from build123d import *

# Parameters (mm, degrees)
SKETCH_1_R      = 1.75
EXTRUDE_1_DEPTH = 3
FILLET_3_R      = 5


with BuildPart() as part:
    # 草图1 → 凸台-拉伸1 (new body)
    with BuildSketch(Plane(origin=(0, 0, 0), x_dir=(1, 0, 0), z_dir=(0, 1, 0))):
        with BuildLine():
            Line((-27.5, -18.562205506), (-37.85023308, -27.436866757))
            ThreePointArc((-37.85023308, -27.436866757), (-39.59101252, -31.447551796), (-37.512145027, -35.293876989))
            Line((-37.512145027, -35.293876989), (-26.035533906, -43.535533906))
            ThreePointArc((-26.035533906, -43.535533906), (-24.413417162, -44.619397663), (-22.5, -45))
            Line((-22.5, -45), (-22.5, -54))
            ThreePointArc((-22.5, -54), (-21.914213562, -55.414213562), (-20.5, -56))
            Line((-20.5, -56), (-16.5, -56))
            ThreePointArc((-16.5, -56), (-15.085786438, -55.414213562), (-14.5, -54))
            Line((-14.5, -54), (-14.5, -45))
            Line((-14.5, -45), (14.5, -45))
            Line((14.5, -45), (14.5, -54))
            ThreePointArc((14.5, -54), (15.085786438, -55.414213562), (16.5, -56))
            Line((16.5, -56), (20.5, -56))
            ThreePointArc((20.5, -56), (21.914213562, -55.414213562), (22.5, -54))
            Line((22.5, -54), (22.5, -45))
            ThreePointArc((22.5, -45), (24.413417162, -44.619397663), (26.035533906, -43.535533906))
            Line((26.035533906, -43.535533906), (37.512145027, -35.293876989))
            ThreePointArc((37.512145027, -35.293876989), (39.59101252, -31.447551796), (37.85023308, -27.436866757))
            Line((37.85023308, -27.436866757), (27.5, -18.562205506))
            Line((27.5, -18.562205506), (27.5, 18.562205506))
            Line((27.5, 18.562205506), (37.85023308, 27.436866757))
            ThreePointArc((37.85023308, 27.436866757), (39.59101252, 31.447551796), (37.512145027, 35.293876989))
            Line((37.512145027, 35.293876989), (26.035533906, 43.535533906))
            ThreePointArc((26.035533906, 43.535533906), (24.413417162, 44.619397663), (22.5, 45))
            Line((22.5, 45), (22.5, 54))
            ThreePointArc((22.5, 54), (21.914213562, 55.414213562), (20.5, 56))
            Line((20.5, 56), (16.5, 56))
            ThreePointArc((16.5, 56), (15.085786438, 55.414213562), (14.5, 54))
            Line((14.5, 54), (14.5, 45))
            Line((14.5, 45), (-14.5, 45))
            Line((-14.5, 45), (-14.5, 54))
            ThreePointArc((-14.5, 54), (-15.085786438, 55.414213562), (-16.5, 56))
            Line((-16.5, 56), (-20.5, 56))
            ThreePointArc((-20.5, 56), (-21.914213562, 55.414213562), (-22.5, 54))
            Line((-22.5, 54), (-22.5, 45))
            ThreePointArc((-22.5, 45), (-24.413417162, 44.619397663), (-26.035533906, 43.535533906))
            Line((-26.035533906, 43.535533906), (-37.512145027, 35.293876989))
            ThreePointArc((-37.512145027, 35.293876989), (-39.59101252, 31.447551796), (-37.85023308, 27.436866757))
            Line((-37.85023308, 27.436866757), (-27.5, 18.562205506))
            Line((-27.5, 18.562205506), (-27.5, -18.562205506))
        make_face()
        with Locations((-22.5, -40)):
            Circle(SKETCH_1_R, mode=Mode.SUBTRACT)
        with Locations((22.5, 40)):
            Circle(SKETCH_1_R, mode=Mode.SUBTRACT)
        with Locations((-35, -31.25)):
            Circle(SKETCH_1_R, mode=Mode.SUBTRACT)
        with Locations((-18.5, -49)):
            Circle(SKETCH_1_R, mode=Mode.SUBTRACT)
        with Locations((18.5, -49)):
            Circle(SKETCH_1_R, mode=Mode.SUBTRACT)
        with Locations((-35, 31.25)):
            Circle(SKETCH_1_R, mode=Mode.SUBTRACT)
        with Locations((35, -31.25)):
            Circle(SKETCH_1_R, mode=Mode.SUBTRACT)
        with Locations((-18.5, 49)):
            Circle(SKETCH_1_R, mode=Mode.SUBTRACT)
        with Locations((35, 31.25)):
            Circle(SKETCH_1_R, mode=Mode.SUBTRACT)
        with Locations((18.5, 49)):
            Circle(SKETCH_1_R, mode=Mode.SUBTRACT)
    extrude(amount=EXTRUDE_1_DEPTH)

    # 圆角3
    fillet_3_edges = [part.edges().sort_by_distance(p)[0] for p in [
        (-22.5, 1.5, -45),
        (-14.5, 1.5, -45),
        (14.5, 1.5, -45),
        (22.5, 1.5, -45),
        (27.5, 1.5, -18.562205506),
        (27.5, 1.5, 18.562205506),
        (22.5, 1.5, 45),
        (14.5, 1.5, 45),
        (-14.5, 1.5, 45),
        (-22.5, 1.5, 45),
        (-27.5, 1.5, 18.562205506),
        (-27.5, 1.5, -18.562205506),
    ]]
    fillet(fillet_3_edges, radius=FILLET_3_R)


solid = part.part
Read the model definition and answer for the solid it produces. Units are mm, in the model's axes. A direction names the side the tool comes from. Give positions to 0.01 mm unless a question says otherwise; leave off trailing zeros. Write each loop counter-clockwise with the first axis right and the second up, starting at its lowest first coordinate (ties: lowest second). Pieces come first, ordered by that corner, then holes. Notation, with made-up numbers: (-4.5, 78.25) - (25.5, 78.25) arc R26 cw to (25.5, 113.25) - close; hole circle Ø1 at (16, 76). An arc over 180 degrees is marked (long way). Answer in a Markdown table with one row per item. Add a question column.
Item 1: Section C-C, the plane x = 35 is taken. Write down the section's boundary in (y, z), and give its area (3 significant figures).
Item 2: Section A-A, the plane x = -18.5 is taken. Write down the section's boundary in (y, z), and give its area (3 significant figures).
Item 3: Section B-B, the plane z = 40 is taken. Write down the section's boundary in (x, y).
Item 4: A tool of negligible diameter and unlimited length cuts with its end or side. For faces 5 (the face through (13, 1.52, -46.43)), 6 (the face through (27.97, 1.52, 18.38)), 7 (the face through (-14.5, 1, 52)), from which of +Z, -Z, +X, -X, +Y, -Y can it reach the whole face along a straight path? Write none if from no direction.
Item 5: Section D-D, the plane z = -31.25 is taken. Write down the section's boundary in (x, y), and give its area (3 significant figures).
Item 6: Determine the mould class of faces 1 (the face through (21.11, 1.48, -38.94)), 2 (the face through (-31.85, 1.48, 39.36)), 3 (the face through (19, 1, -56)), 4 (the face through (27.945, 1.521, -18.324)) for opening direction Z: pulls with the +Z half, pulls with the -Z half, needs draft (parallel to the pull), parting line crosses it, or undercut.
Item 7: Find the intervals of material crossed by L1, parallel to Z at x = -18.5, y = 1.4; L2, parallel to Z at x = 34.5, y = 0.7; L3, parallel to Z at x = -35, y = 2.15, in increasing order.
Item 8: Flat-ended cylindrical pins translate along their axes: P1, Ø1, axis at y = 2, z = 43, coming from the +X side; P2, Ø1.5, axis at y = 1.5, z = 52, coming from the -X side; P3, Ø0.9, axis at y = 1.5, z = 1.5, coming from the -X side. Find the tip coordinate at first contact, or state that the pin passes through.
Recorded:
| question | item | result |
|---|---|---|
| 1 | outline | (0, -37.1) - (3, -37.1) - (3, -33) - (0, -33) - close; (0, -29.5) - (3, -29.5) - (3, -24.99) - (0, -24.99) - close; (0, 24.99) - (3, 24.99) - (3, 29.5) - (0, 29.5) - close; (0, 33) - (3, 33) - (3, 37.1) - (0, 37.1) - close |
| 1 | area | 51.6 mm2 |
| 2 | outline | (0, -56) - (3, -56) - (3, -50.75) - (0, -50.75) - close; (0, -47.25) - (3, -47.25) - (3, 47.25) - (0, 47.25) - close; (0, 50.75) - (3, 50.75) - (3, 56) - (0, 56) - close |
| 2 | area | 315 mm2 |
| 3 | outline | (-30.96, 0) - (-24.25, 0) - (-24.25, 3) - (-30.96, 3) - close; (-20.75, 0) - (30.96, 0) - (30.96, 3) - (-20.75, 3) - close |
| 4 | face 5 | -Z, +Y, -Y |
| 4 | face 6 | +X, +Y, -Y |
| 4 | face 7 | +Z, +Y, -Y |
| 5 | outline | (-39.6, 0) - (-36.75, 0) - (-36.75, 3) - (-39.6, 3) - close; (-33.25, 0) - (33.25, 0) - (33.25, 3) - (-33.25, 3) - close; (36.75, 0) - (39.6, 0) - (39.6, 3) - (36.75, 3) - close |
| 5 | area | 217 mm2 |
| 6 | face 1 | undercut |
| 6 | face 2 | pulls with the +Z half |
| 6 | face 3 | pulls with the -Z half |
| 6 | face 4 | undercut |
| 7 | L1 | z = -56 to -50.75, -47.25 to 47.25, 50.75 to 56 |
| 7 | L2 | z = -37.46 to -32.93, -29.57 to -24.56, 24.56 to 29.57, 32.93 to 37.46 |
| 7 | L3 | z = -37.1 to -33, -29.5 to -24.99, 24.99 to 29.5, 33 to 37.1 |
| 8 | P1 | stops at x = 27.48 |
| 8 | P2 | stops at x = -22.5 |
| 8 | P3 | stops at x = -27.5 |
